Build history of the part. All positions in model axes, mm. A direction names the side the tool comes from. Round coordinates to 2 decimals unless told otherwise and drop trailing zeros. Write each loop counter-clockwise with the first axis right and the second up, starting at its lowest first coordinate (ties: lowest second). Pieces come first, ordered by that corner, then holes. Notation, with made-up numbers: (-26, 87) -> (2, 87) arc R20 ccw to (2, 95) -> close; hole circle Ø6 at (82.5, 15.5). An arc over 180 degrees is marked (long way). Answer as CSV lines item,"result".
from build123d import *

# Parameters (mm, degrees)
SKETCH1_R               = 3.96875
EXTRUDE1_DEPTH          = 234.95
CHAMFER1_SIZE           = 1.27
SKETCH3_W               = 0.79375
SKETCH3_H               = 6.35
CUT_EXTRUDE1_DEPTH      = 4.96875
CUT_EXTRUDE1_DEPTH_BACK = 4.96875
SKETCH4_W               = 0.79375
SKETCH4_H               = 190.5


with BuildPart() as part:
    # Sketch1 → Extrude1 (new body)
    with BuildSketch(Plane.XY):
        Circle(SKETCH1_R)
    extrude(amount=EXTRUDE1_DEPTH)

    # Chamfer1
    chamfer1_edges = [part.edges().sort_by_distance(p)[0] for p in [
        (-3.96875, 0, 0),
        (-3.96875, 0, 234.95),
    ]]
    chamfer(chamfer1_edges, length=CHAMFER1_SIZE)

    # Sketch3 → Cut-Extrude1 (cut, two sides)
    with BuildSketch(Plane(origin=(0, 0, 0), x_dir=(1, 0, 0), z_dir=(0, 1, 0))) as cut_extrude1_sk:
        with Locations((3.571875, -231.775)):
            Rectangle(SKETCH3_W, SKETCH3_H)
        with Locations((-3.571875, -231.775)):
            Rectangle(SKETCH3_W, SKETCH3_H)
    extrude(amount=CUT_EXTRUDE1_DEPTH, mode=Mode.SUBTRACT)
    extrude(cut_extrude1_sk.sketch, amount=-CUT_EXTRUDE1_DEPTH_BACK, mode=Mode.SUBTRACT)

    # Sketch4 → Revolve1 (revolve)
    with BuildSketch(Plane(origin=(0, 0, 0), x_dir=(1, 0, 0), z_dir=(0, 1, 0)), mode=Mode.PRIVATE) as revolve1_sk:
        with Locations((-4.365625, -117.475)):
            Rectangle(SKETCH4_W, SKETCH4_H)
    revolve(revolve1_sk.sketch.rotate(Axis((0, 0, -16.320632547), (0, 0, 1)), 323.130102354), axis=Axis((0, 0, -16.320632547), (0, 0, 1)))  # turned: the seam where the file's is


solid = part.part
1. Which spindle directions (+Z, -Z, +X, -X, +Y, -Y) get a long thin tool onto all of the face, cutting with end or side? Do faces 1 (the flat face through (-1, -4, 212.725)), 2 (the flat face through (0, 0, 0)), 3 (the cylindrical face through (3.666, -1.52, 11.601)), 4 (the flat face through (3.175, 0, 232)), 5 (the flat face through (-3.175, 0, 232)). Say none if no direction does.
Results found:
face 1,"+Z"
face 2,"-Z, +X, -X, +Y, -Y"
face 3,"-Z"
face 4,"+Z, +X, +Y, -Y"
face 5,"+Z, -X, +Y, -Y"
2. Cut at C-C, the plane z = 106.5. Write the cut outline in (x, y) (1 decimal).
Results found:
outline,"circle Ø9.5 at (0, 0)"
3. Drop flat-ended pins along their axis: pin 1 Ø5 at (y, z) = (-0.5, 232) entering from -X (3 decimals); pin 2 Ø1.5 at (x, y) = (1.5, 3.5) entering from +Z; pin 3 Ø0.9 at (x, y) = (-3.5, -1) entering from +Z. Give the stop position or say it passes through.
Results found:
pin 1,"stops at x = -3.175"
pin 2,"stops at z = 234.59"
pin 3,"stops at z = 234.46"
4. Probe line 1 along X through (y, z) = (0.25, 89.5); line 2 along Y through (x, z) = (0.5, 167.5); line 3 along Z through (x, y) = (3.75, -2.25) (3 decimals). List the from-to ranges inside material, lowest first.
Results found:
line 1,"x = -4.76 to 4.76"
line 2,"y = -4.74 to 4.74"
line 3,"z = 22.225 to 212.725"
